```python
from build123d import *

# Parameters (mm, degrees)
FILLET_R    = 0.4
FILLET002_R = 0.2
FILLET003_R = 0.2


with BuildPart() as inner_cutout:
    # Cone → Cone (revolve)
    with BuildSketch(Plane.XZ):
        Polygon((0, 0), (2, 0), (1.75, 30), (0, 30), align=None)
    revolve(axis=Axis((0, 0, 0), (0, 0, 1)))


with BuildPart() as fillet003:
    # Cone001 → Cone001 (revolve)
    with BuildSketch(Plane.XZ):
        Polygon((0, 0), (4, 0), (3.75, 30), (0, 30), align=None)
    revolve(axis=Axis((0, 0, 0), (0, 0, 1)))

    # Cut: cut Inner Cutout
    add(inner_cutout.part, mode=Mode.SUBTRACT)

    # Fillet
    fillet_edges = [fillet003.edges().sort_by_distance(p)[0] for p in [
        (-3.75, 0, 30),
    ]]
    fillet(fillet_edges, radius=FILLET_R)

    # Fillet002
    fillet002_edges = [fillet003.edges().sort_by_distance(p)[0] for p in [
        (-4, 0, 0),
    ]]
    fillet(fillet002_edges, radius=FILLET002_R)

    # Fillet003
    fillet003_edges = [fillet003.edges().sort_by_distance(p)[0] for p in [
        (-2, 0, 0),
    ]]
    fillet(fillet003_edges, radius=FILLET003_R)


solid = fillet003.part
```
Geometry check sheet. Reference: the model listing, model coordinates, mm. Give positions to 0.01 mm unless a question says otherwise; leave off trailing zeros. Order: outer loops, then holes, each group sorted by start corner. A loop starts at its lowest first (then second) coordinate and runs counter-clockwise, first axis right, second up. Notation, with made-up numbers: (-15, 82) -> (17, 82) arc R21 ccw to (17, 96) -> close; hole circle Ø7 at (5.5, 40). An arc over 180 degrees is marked (long way). Write each question's results on one line, items separated by ' | '. Start each with the question number.
(1) Scan lines: line 1 (Y direction, x = -0.5, z = 9.5); line 2 (X direction, y = 0, z = 21) (3 decimals); line 3 (Y direction, x = -0.5, z = 23). Record each from-to range of solid material in increasing order.
(2) Sectioned sample at A-A (z = 6). Enter the section's corners in (x, y), plus the area to 3 significant figures.
(3) Gauge pin test, flat ends, axial feed: P1, Ø1.5, axis at x = 0, y = -0.5, coming from the -Z side; P2, Ø1, axis at x = 2, z = 10.5, coming from the -Y side; P3, Ø3, axis at y = 3, z = 17.5, coming from the -X side; P4, Ø4, axis at x = 1, y = -2.5, coming from the -Z side. Record the tip position at first contact, or that the pin passes through.
(4) Mould release check, pull along X, two halves, no side actions. Record for faces 1 (the face through (-2, -2, 0)), 2 (the face through (-0.406, -1.828, 15.308)), 3 (the face through (-0.5, 3.84, 15.11)): pulls with the +X half, pulls with the -X half, needs draft (parallel to the pull), parting line crosses it, or undercut.
(5) Sectioned sample at B-B (z = 25.5). Enter the section's corners in (x, y) (1 decimal).
Answer below:
1) line 1: -3.89 to -1.85, 1.85 to 3.89 | line 2: -3.825 to -1.825, 1.825 to 3.825 | line 3: -3.78 to -1.74, 1.74 to 3.78
2) outline: circle Ø7.9 at (0, 0); hole circle Ø3.9 at (0, 0) | area: 37.1 mm2
3) P1: through | P2: y = -3.61 | P3: x = -3.55 | P4: z = 0
4) face 1: needs draft | face 2: undercut | face 3: parting line crosses it
5) outline: circle Ø7.6 at (0, 0); hole circle Ø3.6 at (0, 0)
